Verification items for the finished model (mm, model axes). A direction names the side the tool comes from. Give positions to 0.01 mm unless a question says otherwise; leave off trailing zeros. Order: outer loops, then holes, each group sorted by start corner. A loop starts at its lowest first (then second) coordinate and runs counter-clockwise, first axis right, second up.
(1) Mould release check, pull along Z, two halves, no side actions. Record for faces 1 (the face through (0, 20.75, 14)), 2 (the face through (-18.527, -18.258, 25.336)), 3 (the face through (-0.1, -2.4, -2)): pulls with the +Z half, pulls with the -Z half, needs draft (parallel to the pull), parting line crosses it, or undercut.
(2) Sectioned sample at A-A on x = 0. Record the cut outline in (y, z), plus the area to 3 significant figures.
(3) Sectioned sample at D-D on y = 8. Record the cut outline in (x, z), plus the area to 3 significant figures.
(4) Scan lines: L1, parallel to Y at x = 15.5, z = 3.25; L2, parallel to X at y = -15, z = 1. Record each from-to range of solid material in increasing order.
(5) Access from +Z, -Z, +X, -X, +Y, -Y to the whole of each face (thin tool, end or side, straight path). Record for faces 4 (the face through (0, -20.75, 14)), 5 (the face through (-15, 16, 10)), 6 (the face through (20.75, 0, 14)).
(6) Sectioned sample at C-C on x = -6. Record the cut outline in (y, z).
(7) Gauge pin test, flat ends, axial feed: pin 1 (3.5 mm diameter, centred on x = -15.5, y = 15.5, fed in from -Z); pin 2 (12.5 mm diameter, centred on x = -7, y = 6.5, fed in from -Z); pin 3 (4 mm diameter, centred on y = 2, z = 14, fed in from +X). Record the tip position at first contact, or that the pin passes through.
```python
from build123d import *

# Parameters (mm, degrees)
RESSALTO_EXTRUS_O1_DEPTH   = 30
CORTE_EXTRUS_O_FINA1_START = -22.8
CORTE_EXTRUS_O_FINA1_DEPTH = 13.6
ESBO_O3_R                  = 2.25
RESSALTO_EXTRUS_O2_DEPTH   = 20
ESBO_O4_R                  = 10
RESSALTO_EXTRUS_O3_DEPTH   = 2
ESBO_O5_R                  = 1.5
CORTE_EXTRUS_O1_DEPTH      = 10


# Read off the part's stored shape, not the designer's step: Corte-Extrusão-Fina1
with BuildPart() as part:
    # Esboço1 → Ressalto-extrusão1 (new body)
    with BuildSketch(Plane.XY):
        Polygon((-21, -15.592171873), (-15.984175996, -21), (15.592171873, -21), (21, -15.984175996), (21, 15.592171873), (15.984175996, 21), (-15.592171873, 21), (-21, 15.984175996), align=None)
    extrude(amount=RESSALTO_EXTRUS_O1_DEPTH)

    # Corte-Extrusão-Fina1 outline → Corte-Extrusão-Fina1 (cut)
    with BuildSketch(Plane.XY.offset(30).offset(CORTE_EXTRUS_O_FINA1_START)):
        Polygon((15.592171873, -21), (21, -15.984175996), (21, 15.592171873), (15.984175996, 21), (-15.592171873, 21), (-21, 15.984175996), (-21, -15.592171873), (-15.984175996, -21), align=None)
        Polygon((14.605339059, 20.75), (20.75, 14.605339059), (20.75, -14.605339059), (14.605339059, -20.75), (-14.605339059, -20.75), (-20.75, -14.605339059), (-20.75, 14.605339059), (-14.605339059, 20.75), align=None, mode=Mode.SUBTRACT)
    extrude(amount=CORTE_EXTRUS_O_FINA1_DEPTH, mode=Mode.SUBTRACT)

    # Esboço3 → Ressalto-extrusão2 (add)
    with BuildSketch(Plane(origin=(0, 0, 0), x_dir=(-1, 0, 0), z_dir=(0, 0, -1))):
        with Locations(Location((0, 0, 0), (0, 0, 180))):
            Circle(ESBO_O3_R)
    extrude(amount=RESSALTO_EXTRUS_O2_DEPTH)

    # Esboço4 → Ressalto-extrusão3 (add)
    with BuildSketch(Plane(origin=(0, 0, 0), x_dir=(-1, 0, 0), z_dir=(0, 0, -1))):
        with Locations(Location((0, 0, 0), (0, 0, 180))):
            Circle(ESBO_O4_R)
    extrude(amount=RESSALTO_EXTRUS_O3_DEPTH)

    # Esboço5 → Corte-extrusão1 (cut)
    with BuildSketch(Plane(origin=(0, 0, 0), x_dir=(-1, 0, 0), z_dir=(0, 0, -1))):
        with Locations((15.5, -15.5)):
            Circle(ESBO_O5_R)
        with Locations((-15.5, -15.5)):
            Circle(ESBO_O5_R)
        with Locations((-15.5, 15.5)):
            Circle(ESBO_O5_R)
        with Locations((15.5, 15.5)):
            Circle(ESBO_O5_R)
    extrude(amount=-CORTE_EXTRUS_O1_DEPTH, mode=Mode.SUBTRACT)


solid = part.part
```
Ans:
1. face 1: undercut
1. face 2: needs draft
1. face 3: pulls with the -Z half
2. outline: (-21, 0) - (-10, 0) - (-10, -2) - (-2.25, -2) - (-2.25, -20) - (2.25, -20) - (2.25, -2) - (10, -2) - (10, 0) - (21, 0) - (21, 7.2) - (20.75, 7.2) - (20.75, 20.8) - (21, 20.8) - (21, 30) - (-21, 30) - (-21, 20.8) - (-20.75, 20.8) - (-20.75, 7.2) - (-21, 7.2) - close
2. area: 1,370 mm2
3. outline: (-21, 0) - (-6, 0) - (-6, -2) - (6, -2) - (6, 0) - (21, 0) - (21, 7.2) - (20.75, 7.2) - (20.75, 20.8) - (21, 20.8) - (21, 30) - (-21, 30) - (-21, 20.8) - (-20.75, 20.8) - (-20.75, 7.2) - (-21, 7.2) - close
3. area: 1,280 mm2
4. L1: y = -21 to -17, -14 to 14, 17 to 21
4. L2: x = -21 to -16.91, -14.09 to 14.09, 16.91 to 21
5. face 4: +X, -X, -Y
5. face 5: -Z
5. face 6: +X, +Y, -Y
6. outline: (-21, 0) - (-8, 0) - (-8, -2) - (8, -2) - (8, 0) - (21, 0) - (21, 7.2) - (20.75, 7.2) - (20.75, 20.8) - (21, 20.8) - (21, 30) - (-21, 30) - (-21, 20.8) - (-20.75, 20.8) - (-20.75, 7.2) - (-21, 7.2) - close
7. pin 1: stops at z = 0
7. pin 2: stops at z = -2
7. pin 3: stops at x = 20.75
